from build123d import *

# Parameters (mm, degrees)
F0_R     = 3.175
F1_DEPTH = 12.7
F2_W     = 5.08
F2_H     = 10.16
F3_DEPTH = 25.401
F4_R     = 1.27


with BuildPart() as f1:
    # F0 (on Front) → F1 (new body)
    with BuildSketch(Plane.XZ):
        Polygon((12.7, 12.7), (0, 0), (25.4, 0), align=None)
        with Locations((12.7, 6.35)):
            Circle(F0_R, mode=Mode.SUBTRACT)
    extrude(amount=F1_DEPTH)

    # F2 (on Right) → F3 (cut, through all)
    with BuildSketch(Plane.YZ):
        with Locations((-6.35, 7.62)):
            Rectangle(F2_W, F2_H)
    extrude(amount=F3_DEPTH, mode=Mode.SUBTRACT)

    # F4
    f4_edges = [f1.edges().sort_by_distance(p)[0] for p in [
        (12.7, -10.795, 12.7),
        (12.7, -1.905, 12.7),
        (0, -6.35, 0),
        (25.4, -6.35, 0),
    ]]
    fillet(f4_edges, radius=F4_R)


solid = f1.part
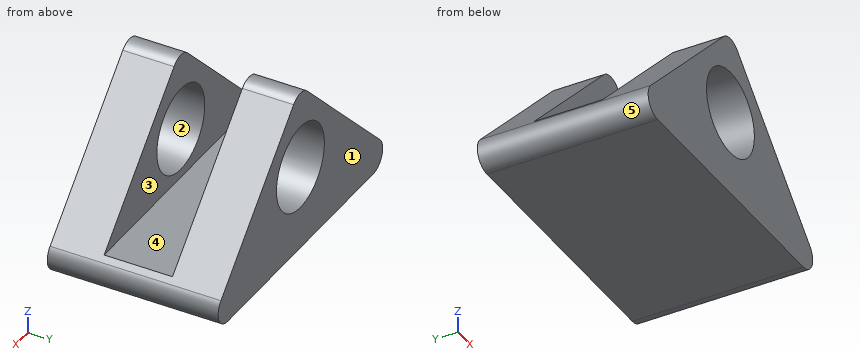
Input: part model. Units: mm. Frame: model coordinates. Face numbers are marked on the shaded views. A direction names the side the tool comes from. Coordinates: 2 decimals unless noted, no trailing zeros. Loops run counter-clockwise (first coordinate to the right, second up) from the corner with the lowest first, then second, coordinate; pieces in that order, holes last. Notation, with made-up numbers: (51, 80) -> (76, 80) arc R16 cw to (76, 97) -> close; hole circle Ø1 at (7, 26.25). An arc over 180 degrees is marked (long way). One line per item, written item: value.
(1) Cut plane B-B (z = 6.35). Output: boundary loops of the cut face in (x, y) (3 decimals), then the cut area to 3 significant figures.
Answer below:
outline: (6.35, -12.7) -> (9.525, -12.7) -> (9.525, -8.89) -> (6.35, -8.89) -> close; (6.35, -3.81) -> (9.525, -3.81) -> (9.525, 0) -> (6.35, 0) -> close; (15.875, -12.7) -> (19.05, -12.7) -> (19.05, -8.89) -> (15.875, -8.89) -> close; (15.875, -3.81) -> (19.05, -3.81) -> (19.05, 0) -> (15.875, 0) -> close
area: 48.4 mm2
(2) Cut plane C-C (x = 18.75). Output: boundary loops of the cut face in (y, z).
Answer below:
outline: (-12.7, 0) -> (0, 0) -> (0, 6.65) -> (-3.81, 6.65) -> (-3.81, 2.54) -> (-8.89, 2.54) -> (-8.89, 6.65) -> (-12.7, 6.65) -> close
(3) Pin query (flat end, axial travel): pin 1 Ø1 at (y, z) = (-11, 10.5) entering from +X; pin 2 Ø1.5 at (x, y) = (14, -7) entering from +Z; pin 3 Ø5.5 at (x, z) = (12.7, 6.35) entering from -Y; pin 4 Ø5 at (y, z) = (-7, 9) entering from -X. Return the tip coordinate at first contact, or that it passes through.
Answer below:
pin 1: stops at x = 15.4
pin 2: stops at z = 2.54
pin 3: passes through
pin 4: stops at x = 7.36
(4) Ray query, line 1 along Z through (x, y) = (12.7, -1.5) (3 decimals); line 2 along Y through (x, z) = (18, 3); line 3 along Z through (x, y) = (15.25, -3.5). Return the intervals inside material, ascending.
Answer below:
line 1: z = 0 to 3.175, 9.525 to 12.174
line 2: y = -12.7 to -8.89, -3.81 to 0
line 3: z = 0 to 4.46, 8.24 to 10.15
(5) Cut plane D-D (y = -10.5). Output: boundary loops of the cut face in (x, z) (3 decimals).
Answer below:
outline: (2.168, 2.168) arc R1.27 ccw to (3.066, 0) -> (22.334, 0) arc R1.27 ccw to (23.232, 2.168) -> (13.598, 11.802) arc R1.27 ccw to (11.802, 11.802) -> close; hole circle Ø6.35 at (12.7, 6.35)
(6) Cut plane A-A (z = 10). Output: boundary loops of the cut face in (x, y), then the cut area to 3 significant figures.
Answer below:
outline: (10, -12.7) -> (15.4, -12.7) -> (15.4, -8.89) -> (10, -8.89) -> close; (10, -3.81) -> (15.4, -3.81) -> (15.4, 0) -> (10, 0) -> close
area: 41.1 mm2
(7) Set-up query: the marked faces 4 and 5. Return all of +Z, -Z, +X, -X, +Y, -Y with unobstructed straight access to the full face (end or side cutting, diameter ignored); none if empty.
Answer below:
face 4: +Z, +X, -X
face 5: -X, +Y, -Y
(8) Draft query along Y for the marked faces 1, 2 and 3. Return one class per face: pulls with the +Y half, pulls with the -Y half, needs draft (parallel to the pull), parting line crosses it, or undercut.
Answer below:
face 1: pulls with the +Y half
face 2: needs draft
face 3: undercut
